Verification items for this drawing (mm, ordinates from the low corner). A direction names the side the tool comes from. Give positions to 0.01 mm unless a question says otherwise; leave off trailing zeros. Write each loop counter-clockwise with the first axis right and the second up, starting at its lowest first coordinate (ties: lowest second). Pieces come first, ordered by that corner, then holes. Notation, with made-up numbers: (-29.5, 50) -> (-19.5, 50) arc R15 ccw to (-19.5, 59) -> close; hole circle Ø9 at (5, 66). An arc over 180 degrees is marked (long way). One line per item, written item: value.
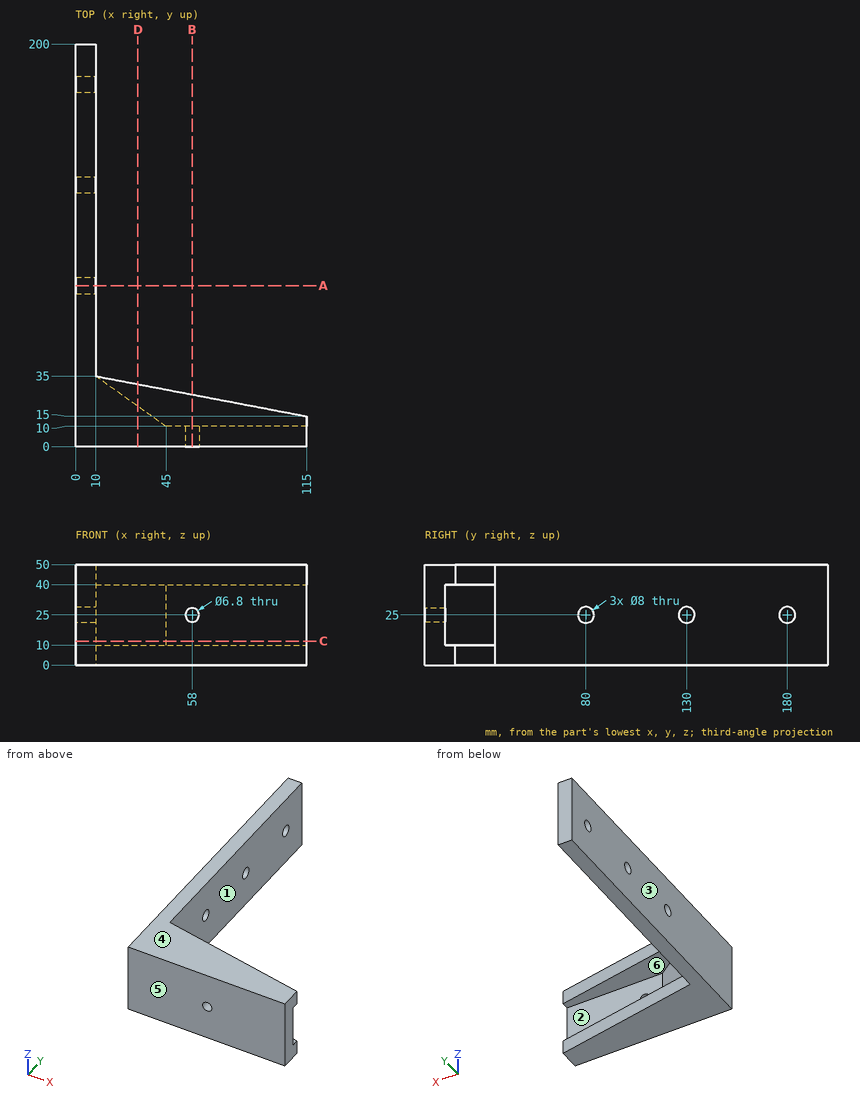
1) Scan lines: probe 1 along Y at (x, z) = (7, 25); probe 2 along Y at (x, z) = (47.5, 25). Record each from-to range of solid material in increasing order.
Verdict:
probe 1: 0 to 76, 84 to 126, 134 to 176, 184 to 200
probe 2: 0 to 10
2) Sectioned sample at D-D on x = 31. Record the cut outline in (y, z).
Verdict:
outline: (0, 0) -> (31, 0) -> (31, 10) -> (20, 10) -> (20, 40) -> (31, 40) -> (31, 50) -> (0, 50) -> close
3) Depth check by flat-ended pin: pin 1 Ø10.5 at (y, z) = (180, 25) entering from +X; pin 2 Ø8 at (x, z) = (58, 25) entering from +Y; pin 3 Ø5 at (y, z) = (80, 25) entering from +X. Enter the tip coordinate at first touch or a pass-through.
Verdict:
pin 1: x = 10
pin 2: y = 10
pin 3: through
4) Sectioned sample at A-A on y = 80. Record the cut outline in (x, z).
Verdict:
outline: (0, 0) -> (10, 0) -> (10, 21) -> (0, 21) -> close; (0, 29) -> (10, 29) -> (10, 50) -> (0, 50) -> close
5) Tool access check on the marked faces 1, 2 and 3. Record the directions out of +Z, -Z, +X, -X, +Y, -Y that give a thin tool (end or side, any length) a straight path to the whole face; none if there is none.
Verdict:
face 1: +Z, -Z, +X, +Y
face 2: +X, +Y
face 3: +Z, -Z, -X, +Y, -Y
6) Sectioned sample at C-C on z = 12. Record the cut outline in (x, y), plus the area to 3 significant figures.
Verdict:
outline: (0, 0) -> (115, 0) -> (115, 10) -> (45, 10) -> (10, 35) -> (10, 200) -> (0, 200) -> close
area: 3,490 mm^2
7) Sectioned sample at B-B on x = 58. Record the cut outline in (y, z).
Verdict:
outline: (0, 0) -> (25.86, 0) -> (25.86, 10) -> (10, 10) -> (10, 21.6) -> (0, 21.6) -> close; (0, 28.4) -> (10, 28.4) -> (10, 40) -> (25.86, 40) -> (25.86, 50) -> (0, 50) -> close
8) Mould release check, pull along Z, two halves, no side actions. Record for the marked faces 4, 5 and 6: released by +Z, released by -Z, zero draft, split by the parting line, or undercut.
Verdict:
face 4: released by +Z
face 5: zero draft
face 6: undercut
